from build123d import *

# Parameters (mm, degrees)
F0_R     = 6.35
F1_DEPTH = 50.8
F2_W     = 101.6
F2_H     = 25.4
F3_DEPTH = 203.2
F4_W     = 76.2
F4_H     = 190.5
F5_DEPTH = 50.8


with BuildPart() as f1:
    # F0 (on Top) → F1 (new body)
    with BuildSketch(Plane.XY):
        Polygon((247.65, 38.1), (-247.65, 38.1), (-247.65, -38.1), (171.45, -38.1), (171.45, -63.5), (95.25, -63.5), (95.25, -311.15), (171.45, -311.15), (171.45, -1181.1), (247.65, -1181.1), (247.65, -311.15), (323.85, -311.15), (323.85, -63.5), (247.65, -63.5), (247.65, -38.1), align=None)
        with Locations((82.55, 0)):
            Circle(F0_R, mode=Mode.SUBTRACT)
    extrude(amount=F1_DEPTH)

    # F2 (on face) → F3 (join)
    with BuildSketch(Plane.XY.offset(50.8)):
        with Locations((-196.85, -25.4)):
            Rectangle(F2_W, F2_H)
    extrude(amount=F3_DEPTH)

    # F4 (on face) → F5 (cut)
    with BuildSketch(Plane.XY.offset(50.8)):
        with Locations((209.55, -183.31946)):
            Rectangle(F4_W, F4_H)
    extrude(amount=-F5_DEPTH, mode=Mode.SUBTRACT)


solid = f1.part
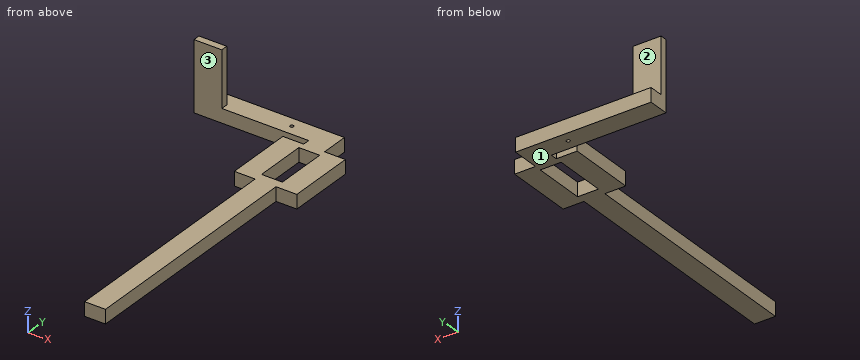
Geometry check sheet. Reference: the model listing, model coordinates, mm. Face numbers are marked on the shaded views. A direction names the side the tool comes from. Round coordinates to 2 decimals unless told otherwise and drop trailing zeros. Order: outer loops, then holes, each group sorted by start corner. A loop starts at its lowest first (then second) coordinate and runs counter-clockwise, first axis right, second up. Notation, with made-up numbers: (-26.75, 44) - (25.25, 44) arc R31 cw to (25.25, 83) - close; hole circle Ø1 at (-26.75, -15). An arc over 180 degrees is marked (long way). One line per question, with ' | ' between items. Start each with the question number.
(1) Sectioned sample at C-C on z = 146. Record the cut outline in (x, y).
(2) Sectioned sample at D-D on y = -715. Record the cut outline in (x, z), and give its area (3 significant figures).
(3) Sectioned sample at B-B on x = -202. Record the cut outline in (y, z), and give its area (3 significant figures).
(4) Thickness scan on L1, parallel to Y at x = 82.55, z = 32.5; L2, parallel to X at y = -187, z = 38.5; L3, parallel to Z at x = 173.5, y = -1013.5. Record the ranges inside material, lowest first. Write a range as [from, to].
(5) Sectioned sample at A-A on x = 215.5. Record the cut outline in (y, z), and give its area (3 significant figures).
(6) Access from +Z, -Z, +X, -X, +Y, -Y to the whole of each face (thin tool, end or side, straight path). Record for the marked faces 1, 2 and 3.
(7) Depth check by flat-ended pin: pin 1 Ø12 at (y, z) = (-797, 46.5) entering from +X; pin 2 Ø7.5 at (y, z) = (-52.5, 14.5) entering from -X; pin 3 Ø7.5 at (y, z) = (-29, 194) entering from +X. Enter the tip coordinate at first touch or a pass-through.
Conclusion:
1) outline: (-247.65, -38.1) - (-146.05, -38.1) - (-146.05, -12.7) - (-247.65, -12.7) - close
2) outline: (171.45, 0) - (247.65, 0) - (247.65, 50.8) - (171.45, 50.8) - close | area: 3,870 mm2
3) outline: (-38.1, 0) - (38.1, 0) - (38.1, 50.8) - (-12.7, 50.8) - (-12.7, 254) - (-38.1, 254) - close | area: 9,030 mm2
4) L1: y = [-38.1, -6.35], [6.35, 38.1] | L2: x = [95.25, 171.45], [247.65, 323.85] | L3: z = [0, 50.8]
5) outline: (-1181.1, 0) - (-278.57, 0) - (-278.57, 50.8) - (-1181.1, 50.8) - close; (-88.07, 0) - (38.1, 0) - (38.1, 50.8) - (-88.07, 50.8) - close | area: 52,300 mm2
6) face 1: -Z, +X, -X, +Y, -Y | face 2: +Z, +X, -X, +Y | face 3: +Z, -Z, -X
7) pin 1: stops at x = 247.65 | pin 2: stops at x = 171.45 | pin 3: stops at x = -146.05
